Drawing for the job (mm, zero at the part's lowest x, y, z). A direction names the side the tool comes from. Round coordinates to 2 decimals unless told otherwise and drop trailing zeros. Write each loop counter-clockwise with the first axis right and the second up, starting at its lowest first coordinate (ties: lowest second). Pieces come first, ordered by that corner, then holes. Notation, with made-up numbers: M 4.5,87 L 42.5,87 A7 ccw 42.5,99 Z; hole C 44.5,-29.75 d1. An arc over 180 degrees is marked long. Use a Markdown table: item, result.
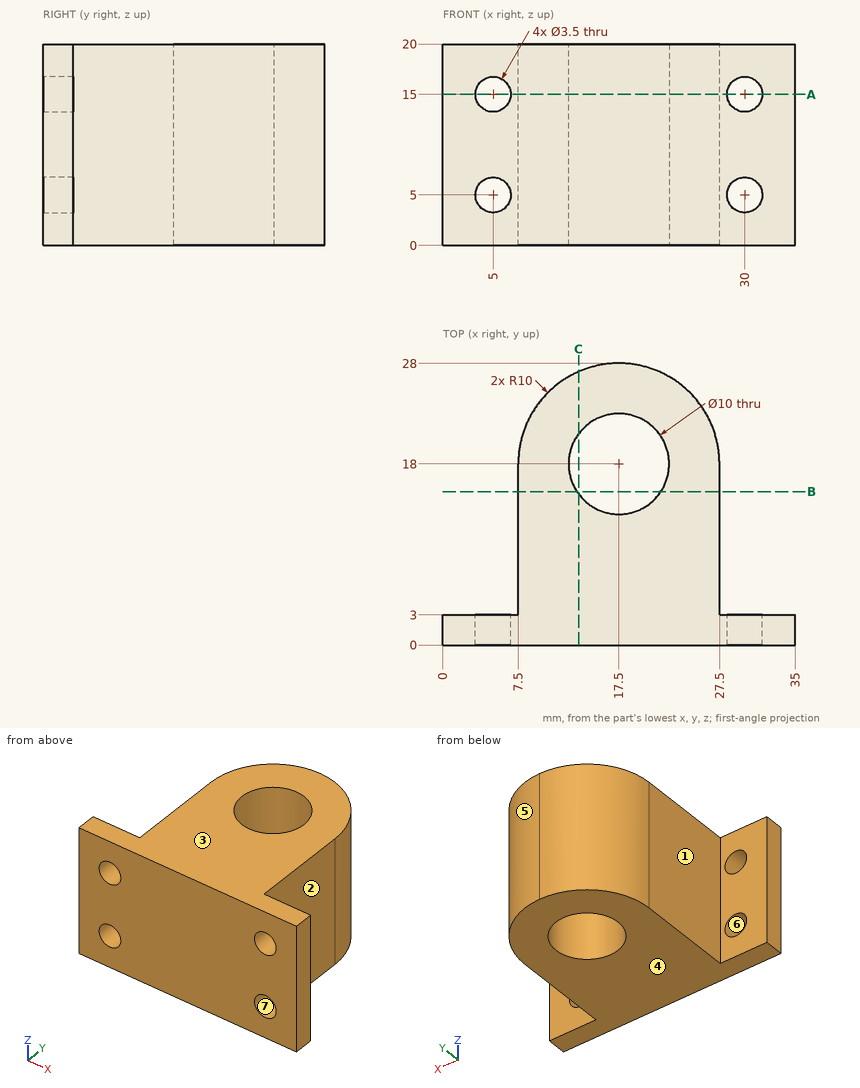
Q1. Cut at B-B on y = 15.25. Give the cut face in (x, z).
Response values:
| item | result |
|---|---|
| outline | M 7.5,0 L 13.32,0 L 13.32,20 L 7.5,20 Z; M 21.68,0 L 27.5,0 L 27.5,20 L 21.68,20 Z |
Q2. Which spindle directions (+Z, -Z, +X, -X, +Y, -Y) get a long thin tool onto all of the face, cutting with end or side? Do the marked faces 1, 2 and 3. Say none if no direction does.
Response values:
| item | result |
|---|---|
| face 1 | +Z, -Z, -X, +Y |
| face 2 | +Z, -Z, +X, +Y |
| face 3 | +Z, +X, -X, +Y, -Y |
Q3. Two-plate mould, pull along Z, no slides. Class the marked faces 4, 5, 6 and 7: +Z half, -Z half, draft (parallel to the pull), parting line (faces both ways), or undercut.
Response values:
| item | result |
|---|---|
| face 4 | -Z half |
| face 5 | draft |
| face 6 | undercut |
| face 7 | undercut |
Q4. Drill centre lines: L1, parallel to X at y = 2.35, z = 5; L2, parallel to X at y = 12, z = 11; L3, parallel to Y at x = 13, z = 7. Where is each one in solid material? Low to high.
Response values:
| item | result |
|---|---|
| L1 | x = 0 to 3.25, 6.75 to 28.25, 31.75 to 35 |
| L2 | x = 7.5 to 27.5 |
| L3 | y = 0 to 15.82, 20.18 to 26.93 |
Q5. Cut at C-C on x = 13.5. Give the cut face in (y, z) (3 decimals).
Response values:
| item | result |
|---|---|
| outline | M 0,0 L 15,0 L 15,20 L 0,20 Z; M 21,0 L 27.165,0 L 27.165,20 L 21,20 Z |
Q6. Drop flat-ended pins along their axis: P1, Ø1, axis at y = 16.5, z = 13.5, coming from the -X side; P2, Ø5, axis at x = 7.5, z = 14.5, coming from the +Y side; P3, Ø4, axis at x = 31, z = 5, coming from the +Y side. Give the stop position or say it passes through.
Response values:
| item | result |
|---|---|
| P1 | stops at x = 7.5 |
| P2 | stops at y = 24.61 |
| P3 | stops at y = 3 |
Q7. Cut at A-A on z = 15. Count the separate pieces of the cut face and the enclosed holes in it, and give its area (3 significant figures).
Response values:
| item | result |
|---|---|
| separate pieces | 3 |
| enclosed holes | 1 |
| area | 463 mm2 |
